```python
from build123d import *
from build123d.topology import SkipClean

# Parameters (mm, degrees)
SKETCH_1_R                      = 25
EXTRUDE_1_DEPTH                 = 5
CUT_EXTRUDE_1_REACH             = 37.707
SKETCH_2_R                      = 15
SKETCH_3_R                      = 22.5
CUT_EXTRUDE_2_DEPTH             = 3
CUT_EXTRUDE_3_REACH             = 37.482
SKETCH_4_R                      = 1.25
CHAMFER_1_SIZE                  = 1
EXTRUDE_2_DEPTH                 = 1.5
EXTRUDE_3_DEPTH                 = 5
CUT_EXTRUDE_4_REACH             = 41.37
SKETCH_10_W                     = 20
SKETCH_10_H                     = 2
EXTRUDE_START                   = 20
EXTRUDE_4_DEPTH                 = 20
CUT_EXTRUDE_5_REACH             = 60.086
SKETCH_11_R                     = 1.65
CUT_EXTRUDE_5_DIRECTION_2_DEPTH = 59.086142926
CUT_EXTRUDE_6_DEPTH             = 3
CHAMFER_4_SIZE                  = 8
EXTRUDE_8_DEPTH                 = 2
SKETCH_15_W                     = 2.3
SKETCH_15_H                     = 20
EXTRUDE_9_DEPTH                 = 36
CUT_EXTRUDE_8_REACH             = 48.368
SKETCH_14_R                     = 22.5
EXTRUDE_7_DEPTH                 = 20


# Read off the part's stored shape, not the designer's step: 镜向3
with BuildPart() as part:
    # 草图1 → 凸台-拉伸1 (new body)
    with BuildSketch(Plane(origin=(0, 0, 0), x_dir=(1, 0, 0), z_dir=(0, 1, 0))):
        with Locations(Location((0, 0, 0), (0, 0, 270))):
            Circle(SKETCH_1_R)
    extrude(amount=EXTRUDE_1_DEPTH)

    # 草图2 → 切除-拉伸1 (cut, up to next)
    with BuildSketch(Plane(origin=(0, 5, 0), x_dir=(1, 0, 0), z_dir=(0, 1, 0)), mode=Mode.PRIVATE) as cut_extrude_1_sk1:
        with Locations(Location((0, 0, 0), (0, 0, 270))):
            Circle(SKETCH_2_R)
    cut_extrude_1_tool1 = extrude(cut_extrude_1_sk1.sketch, amount=-CUT_EXTRUDE_1_REACH, mode=Mode.PRIVATE) & part.part
    add(cut_extrude_1_tool1.solids().sort_by_distance((0, 5, 0))[0], mode=Mode.SUBTRACT)

    # 草图3 → 切除-拉伸2 (cut)
    with BuildSketch(Plane(origin=(0, 5, 0), x_dir=(1, 0, 0), z_dir=(0, 1, 0))):
        with Locations(Location((0, 0, 0), (0, 0, 270))):
            Circle(SKETCH_3_R)
    extrude(amount=-CUT_EXTRUDE_2_DEPTH, mode=Mode.SUBTRACT)

    # 草图4 → 切除-拉伸3 (cut, up to next)
    with BuildSketch(Plane(origin=(0, 2, 0), x_dir=(1, 0, 0), z_dir=(0, 1, 0)), mode=Mode.PRIVATE) as cut_extrude_3_sk1:
        with Locations(Location((9.25, -16.02146997, 0), (0, 0, 270))):
            Circle(SKETCH_4_R)
    cut_extrude_3_tool1 = extrude(cut_extrude_3_sk1.sketch, amount=-CUT_EXTRUDE_3_REACH, mode=Mode.PRIVATE) & part.part
    # 草图4 → 切除-拉伸3 (cut, up to next)
    with BuildSketch(Plane(origin=(0, 2, 0), x_dir=(1, 0, 0), z_dir=(0, 1, 0)), mode=Mode.PRIVATE) as cut_extrude_3_sk2:
        with Locations(Location((-18.5, 0, 0), (0, 0, 270))):
            Circle(SKETCH_4_R)
    cut_extrude_3_tool2 = extrude(cut_extrude_3_sk2.sketch, amount=-CUT_EXTRUDE_3_REACH, mode=Mode.PRIVATE) & part.part
    # 草图4 → 切除-拉伸3 (cut, up to next)
    with BuildSketch(Plane(origin=(0, 2, 0), x_dir=(1, 0, 0), z_dir=(0, 1, 0)), mode=Mode.PRIVATE) as cut_extrude_3_sk3:
        with Locations(Location((9.25, 16.02146997, 0), (0, 0, 270))):
            Circle(SKETCH_4_R)
    cut_extrude_3_tool3 = extrude(cut_extrude_3_sk3.sketch, amount=-CUT_EXTRUDE_3_REACH, mode=Mode.PRIVATE) & part.part
    add(cut_extrude_3_tool1.solids().sort_by_distance((9.25, 2, 16.02147))[0], mode=Mode.SUBTRACT)
    add(cut_extrude_3_tool2.solids().sort_by_distance((-18.5, 2, 0))[0], mode=Mode.SUBTRACT)
    add(cut_extrude_3_tool3.solids().sort_by_distance((9.25, 2, -16.02147))[0], mode=Mode.SUBTRACT)

    # 倒角1
    chamfer_1_edges = [part.edges().sort_by_distance(p)[0] for p in [
        (0, 2, -22.5),
    ]]
    chamfer(chamfer_1_edges, length=CHAMFER_1_SIZE)

    # 草图7 → 凸台-拉伸2 (add)
    with BuildSketch(Plane(origin=(0, 2, 0), x_dir=(1, 0, 0), z_dir=(0, 1, 0))):
        with BuildLine():
            ThreePointArc((5.137558045, 19.173627652), (0, 19.85), (-5.137558045, 19.173627652))
            ThreePointArc((-5.137558045, 19.173627652), (-6.268928895, 17.214035858), (-4.309337101, 16.082665008))
            ThreePointArc((-4.309337101, 16.082665008), (0, 16.65), (4.309337101, 16.082665008))
            ThreePointArc((4.309337101, 16.082665008), (6.268928895, 17.214035858), (5.137558045, 19.173627652))
        make_face()
        with BuildLine():
            ThreePointArc((19.173627652, 5.137558045), (17.190604265, 9.925), (14.036069607, 14.036069607))
            ThreePointArc((14.036069607, 14.036069607), (11.773327907, 14.036069607), (11.773327907, 11.773327907))
            ThreePointArc((11.773327907, 11.773327907), (14.419322973, 8.325), (16.082665008, 4.309337101))
            ThreePointArc((16.082665008, 4.309337101), (18.042256802, 3.177966251), (19.173627652, 5.137558045))
        make_face()
        with BuildLine():
            ThreePointArc((14.036069607, -14.036069607), (17.190604265, -9.925), (19.173627652, -5.137558045))
            ThreePointArc((19.173627652, -5.137558045), (18.042256802, -3.177966251), (16.082665008, -4.309337101))
            ThreePointArc((16.082665008, -4.309337101), (14.419322973, -8.325), (11.773327907, -11.773327907))
            ThreePointArc((11.773327907, -11.773327907), (11.773327907, -14.036069607), (14.036069607, -14.036069607))
        make_face()
        with BuildLine():
            ThreePointArc((-5.137558045, -19.173627652), (0, -19.85), (5.137558045, -19.173627652))
            ThreePointArc((5.137558045, -19.173627652), (6.268928895, -17.214035858), (4.309337101, -16.082665008))
            ThreePointArc((4.309337101, -16.082665008), (0, -16.65), (-4.309337101, -16.082665008))
            ThreePointArc((-4.309337101, -16.082665008), (-6.268928895, -17.214035858), (-5.137558045, -19.173627652))
        make_face()
        with BuildLine():
            ThreePointArc((-19.173627652, -5.137558045), (-17.190604265, -9.925), (-14.036069607, -14.036069607))
            ThreePointArc((-14.036069607, -14.036069607), (-11.773327907, -14.036069607), (-11.773327907, -11.773327907))
            ThreePointArc((-11.773327907, -11.773327907), (-14.419322973, -8.325), (-16.082665008, -4.309337101))
            ThreePointArc((-16.082665008, -4.309337101), (-18.042256802, -3.177966251), (-19.173627652, -5.137558045))
        make_face()
        with BuildLine():
            ThreePointArc((-14.036069607, 14.036069607), (-17.190604265, 9.925), (-19.173627652, 5.137558045))
            ThreePointArc((-19.173627652, 5.137558045), (-18.042256802, 3.177966251), (-16.082665008, 4.309337101))
            ThreePointArc((-16.082665008, 4.309337101), (-14.419322973, 8.325), (-11.773327907, 11.773327907))
            ThreePointArc((-11.773327907, 11.773327907), (-11.773327907, 14.036069607), (-14.036069607, 14.036069607))
        make_face()
    extrude(amount=EXTRUDE_2_DEPTH)

    # 草图8 → 凸台-拉伸3 (add)
    with BuildSketch(Plane(origin=(0, 0, 0), x_dir=(1, 0, 0), z_dir=(0, 1, 0))):
        with BuildLine():
            Line((0, 25), (30, 25))
            Line((30, 25), (30, -25))
            Line((30, -25), (0, -25))
            ThreePointArc((0, -25), (25, 0), (0, 25))
        make_face()
    extrude(amount=EXTRUDE_3_DEPTH)

    # 草图10 → 切除-拉伸4 (cut, up to next)
    with BuildSketch(Plane(origin=(0, 5, 0), x_dir=(1, 0, 0), z_dir=(0, 1, 0)), mode=Mode.PRIVATE) as cut_extrude_4_sk1:
        with Locations((20, 24)):
            Rectangle(SKETCH_10_W, SKETCH_10_H)
    cut_extrude_4_tool1 = extrude(cut_extrude_4_sk1.sketch, amount=-CUT_EXTRUDE_4_REACH, mode=Mode.PRIVATE) & part.part
    add(cut_extrude_4_tool1.solids().sort_by_distance((20, 5, -24))[0], mode=Mode.SUBTRACT)

    # 草图9 → 凸台-拉伸4 (add)
    with SkipClean():  # the faces are left unmerged after this step: merging them gives an invalid solid
        with BuildSketch(Plane(origin=(0, 5, 0), x_dir=(1, 0, 0), z_dir=(0, 1, 0)).offset(EXTRUDE_START)):
            with BuildLine():
                Line((13.5, 18), (30, 18))
                Line((30, 18), (30, 23))
                Line((30, 23), (10, 23))
                Line((10, 23), (10, 20.155644371))
                ThreePointArc((10, 20.155644371), (11.799330518, 19.157917406), (13.5, 18))
            make_face()
        extrude(amount=-EXTRUDE_4_DEPTH)

    # 草图11 → 切除-拉伸5 (cut, up to next)
    with BuildSketch(Plane.XY.offset(-18), mode=Mode.PRIVATE) as cut_extrude_5_sk1:
        with Locations(Location((17.75, 15, 0), (0, 0, 180))):
            Circle(SKETCH_11_R)
    cut_extrude_5_tool1 = extrude(cut_extrude_5_sk1.sketch, amount=-CUT_EXTRUDE_5_REACH, mode=Mode.PRIVATE) & part.part
    # 草图11 → 切除-拉伸5 (cut, up to next)
    with BuildSketch(Plane.XY.offset(-18), mode=Mode.PRIVATE) as cut_extrude_5_sk2:
        with Locations(Location((25.75, 21, 0), (0, 0, 180))):
            Circle(SKETCH_11_R)
    cut_extrude_5_tool2 = extrude(cut_extrude_5_sk2.sketch, amount=-CUT_EXTRUDE_5_REACH, mode=Mode.PRIVATE) & part.part
    # 草图11 → 切除-拉伸5 (cut, up to next)
    with BuildSketch(Plane.XY.offset(-18), mode=Mode.PRIVATE) as cut_extrude_5_sk3:
        with Locations(Location((25.75, 9, 0), (0, 0, 180))):
            Circle(SKETCH_11_R)
    cut_extrude_5_tool3 = extrude(cut_extrude_5_sk3.sketch, amount=-CUT_EXTRUDE_5_REACH, mode=Mode.PRIVATE) & part.part
    add(cut_extrude_5_tool1.solids().sort_by_distance((17.75, 15, -18))[0], mode=Mode.SUBTRACT)
    add(cut_extrude_5_tool2.solids().sort_by_distance((25.75, 21, -18))[0], mode=Mode.SUBTRACT)
    add(cut_extrude_5_tool3.solids().sort_by_distance((25.75, 9, -18))[0], mode=Mode.SUBTRACT)

    # 草图11 → 切除-拉伸5 direction 2 (cut)
    with SkipClean():  # the faces are left unmerged after this step: merging them gives an invalid solid
        with BuildSketch(Plane.XY.offset(-18)):
            with Locations(Location((17.75, 15, 0), (0, 0, 180))):
                Circle(SKETCH_11_R)
            with Locations(Location((25.75, 21, 0), (0, 0, 180))):
                Circle(SKETCH_11_R)
            with Locations(Location((25.75, 9, 0), (0, 0, 180))):
                Circle(SKETCH_11_R)
        extrude(amount=CUT_EXTRUDE_5_DIRECTION_2_DEPTH, mode=Mode.SUBTRACT)

    # 草图12 → 切除-拉伸6 (cut)
    with SkipClean():  # the faces are left unmerged after this step: merging them gives an invalid solid
        with BuildSketch(Plane.XY.offset(-18)):
            Polygon((28.6, 22.645448267), (25.75, 24.290896534), (22.9, 22.645448267), (22.9, 19.354551733), (25.75, 17.709103466), (28.6, 19.354551733), align=None)
            Polygon((28.6, 10.645448267), (25.75, 12.290896534), (22.9, 10.645448267), (22.9, 7.354551733), (25.75, 5.709103466), (28.6, 7.354551733), align=None)
            Polygon((20.6, 16.645448267), (17.75, 18.290896534), (14.9, 16.645448267), (14.9, 13.354551733), (17.75, 11.709103466), (20.6, 13.354551733), align=None)
        extrude(amount=-CUT_EXTRUDE_6_DEPTH, mode=Mode.SUBTRACT)

    # 倒角4
    # the kernel refuses this chamfer: 8 mm, written as the material it adds along each edge
    with BuildSketch(Plane(origin=(10, 5, -23), x_dir=(-0.9996219169112968, -0.02749587661058638, 0), z_dir=(0, 0, 1))) as chamfer_4_piece_1_section:
        Polygon((CHAMFER_4_SIZE * 0.999621916911, -CHAMFER_4_SIZE * 0.0274958766106), (-CHAMFER_4_SIZE * 0.0274958766106, -CHAMFER_4_SIZE * 0.999621916911), (0, 0), align=None)
    chamfer_4_piece_1 = extrude(amount=23.417819533, mode=Mode.PRIVATE)
    chamfer_4_piece_1 = chamfer_4_piece_1 - Plane(origin=(0, 7.978966695, 0), x_dir=(0, 0, 1), z_dir=(0, 1, 0)) * Cylinder(22.5, 79, mode=Mode.PRIVATE)
    add(chamfer_4_piece_1)
    # the kernel refuses this chamfer: 8 mm, written as the material it takes off along each edge
    with BuildSketch(Plane(origin=(10, 25, -43.573463904), x_dir=(-0.02749587661058627, -0.9996219169112968, 0), z_dir=(0, 0, 1))) as chamfer_4_2_piece_1:
        Polygon((CHAMFER_4_SIZE * 0.999621916911, CHAMFER_4_SIZE * 0.0274958766106), (-CHAMFER_4_SIZE * 0.0274958766106, CHAMFER_4_SIZE * 0.999621916911), (0, 0), align=None)
    extrude(amount=43.991283437, mode=Mode.SUBTRACT)

    # 草图17 → 凸台-拉伸8 (add)
    with BuildSketch(Plane(origin=(0, 0, -23), x_dir=(-1, 0, 0), z_dir=(0, 0, -1))):
        Polygon((-10, 13), (-10, 5), (-2, 5), align=None)
    extrude(amount=EXTRUDE_8_DEPTH)

    # 镜向3
    split(bisect_by=Plane.XY, keep=Keep.BOTTOM)

    # Mirror 3 2: part across plane


with BuildPart() as part_1:
    add(part.part)
    add(part.part.mirror(Plane.XY))

    # 草图15 → 凸台-拉伸9 (add)
    with BuildSketch(Plane.XY.offset(-18)):
        with Locations((21.75, 15)):
            Rectangle(SKETCH_15_W, SKETCH_15_H)
    extrude(amount=EXTRUDE_9_DEPTH)

    # 草图14 → 切除-拉伸8 (cut, up to next)
    with BuildSketch(Plane(origin=(0, 25, 0), x_dir=(1, 0, 0), z_dir=(0, 1, 0)), mode=Mode.PRIVATE) as cut_extrude_8_sk1:
        with Locations(Location((0, 0, 0), (0, 0, 270))):
            Circle(SKETCH_14_R)
    cut_extrude_8_tool1 = extrude(cut_extrude_8_sk1.sketch, amount=-CUT_EXTRUDE_8_REACH, mode=Mode.PRIVATE) & part_1.part
    add(cut_extrude_8_tool1.solids().sort_by_distance((0, 25, 0))[0], mode=Mode.SUBTRACT)

    # 草图16 → 凸台-拉伸7 (add)
    with BuildSketch(Plane(origin=(0, 5, 0), x_dir=(1, 0, 0), z_dir=(0, 1, 0))):
        with BuildLine():
            Line((22.9, 9.049309366), (22.9, -9.049309366))
            ThreePointArc((22.9, -9.049309366), (24.62315983, 0), (22.9, 9.049309366))
        make_face()
    extrude(amount=EXTRUDE_7_DEPTH)


solid = part_1.part
```
For this review, take the finished solid that the model builds, in its own axes (mm). A direction names the side the tool comes from. Give positions to 0.01 mm unless a question says otherwise; leave off trailing zeros.
1) For faces 4 (the face through (24.623, 14.86, 0.13)), 5 (the face through (24.31, 6.54, 19.48)), 6 (the face through (17.23, 2.74, -9.86)), 7 (the face through (20, 12, -23)), 8 (the face through (27.4, 8.93, -21.99)), list the 3-axis set-ups (+Z, -Z, +X, -X, +Y, -Y) from which the entire face can be reached by the end or side of a thin tool; tool diameter is ignored.
2) Take a section at A-A (y = 15). State how many separate pieces and enclosed holes the cut face has, then the cut area to 3 significant figures.
3) The part is to be moulded in two halves that separate along X. For faces 1 (the face through (17.965, 13.364, 21.986)), 2 (the face through (6, 9, -23)), 3 (the face through (15, 13, -18)), say which applies: released by +X, released by -X, zero draft, split by the parting line, or undercut.
4) Wall thickness on line 1 (Y direction, x = 25.75, z = 21.85); line 2 (Z direction, x = 14, y = 15); line 3 (Y direction, x = 27.5, z = -19.5): over which ranges is each line inside the solid? List them lowest first.
5) Insertion check: pin 1 (8.5 mm diameter, centred on x = 15, z = -10.5, fed in from +Y); pin 2 (5.5 mm diameter, centred on x = 17.75, y = 15, fed in from -Z); pin 3 (5 mm diameter, centred on y = 13, z = 14, fed in from +X); pin 4 (12 mm diameter, centred on x = -2, y = 10.5, fed in from +Z). Each pin has a flat end and moves straight along its axis. Give the tip position at first contact, or say it passes through.
Derived:
1. face 4: +X, +Y
1. face 5: none
1. face 6: +Y
1. face 7: -Z, +X, +Y, -Y
1. face 8: -Z
2. separate pieces: 3
2. enclosed holes: 0
2. area: 225 mm2
3. face 1: undercut
3. face 2: released by -X
3. face 3: zero draft
4. line 1: y = 0 to 7.35, 10.65 to 19.35, 22.65 to 25
4. line 2: z = -23 to -18, 18 to 23
4. line 3: y = 0 to 6.72, 11.28 to 18.72, 23.28 to 25
5. pin 1: stops at y = 5
5. pin 2: stops at z = -23
5. pin 3: stops at x = 22.9
5. pin 4: stops at z = 25
